from build123d import *

# Parameters (mm, degrees)
SKETCH3_R               = 27
SKETCH3_R_2             = 25
BOSS_EXTRUDE2_DEPTH     = 20
SKETCH4_W               = 21.394887062
SKETCH4_H               = 30
CUT_EXTRUDE1_DEPTH      = 28
CUT_EXTRUDE1_DEPTH_BACK = 28
SKETCH5_R               = 1.5
BOSS_EXTRUDE3_DEPTH     = 20
FILLET2_R               = 5
SKETCH6_R               = 32.5
BOSS_EXTRUDE4_DEPTH     = 3
SKETCH7_R               = 4
CUT_EXTRUDE2_DEPTH      = 4
SKETCH8_R               = 1.5
CUT_EXTRUDE3_DEPTH      = 4
CHAMFER1_SIZE           = 1
SKETCH9_R               = 3.5
BOSS_EXTRUDE5_DEPTH     = 30


with BuildPart() as part:
    # Sketch3 → Boss-Extrude2 (new body)
    with BuildSketch(Plane.XY):
        Circle(SKETCH3_R)
        Circle(SKETCH3_R_2, mode=Mode.SUBTRACT)
    extrude(amount=BOSS_EXTRUDE2_DEPTH)

    # Sketch4 → Cut-Extrude1 (cut, two sides)
    with BuildSketch(Plane(origin=(0, 0, 0), x_dir=(0, 0, -1), z_dir=(1, 0, 0))) as cut_extrude1_sk:
        with Locations((-13.697443531, 0)):
            Rectangle(SKETCH4_W, SKETCH4_H)
    extrude(amount=CUT_EXTRUDE1_DEPTH, mode=Mode.SUBTRACT)
    extrude(cut_extrude1_sk.sketch, amount=-CUT_EXTRUDE1_DEPTH_BACK, mode=Mode.SUBTRACT)

    # Sketch5 → Boss-Extrude3 (add)
    with BuildSketch(Plane.XY):
        with BuildLine():
            Line((-15.644487847, 19.5), (15.644487847, 19.5))
            ThreePointArc((15.644487847, 19.5), (0, 26.287924728), (-15.644487847, 19.5))
        make_face()
        with Locations((-7.5, 22.007101127)):
            Circle(SKETCH5_R, mode=Mode.SUBTRACT)
        with Locations((7.5, 22.007101127)):
            Circle(SKETCH5_R, mode=Mode.SUBTRACT)
        with BuildLine():
            ThreePointArc((8.529361055, -23.5), (0, -20.838962679), (-8.529361055, -23.5))
            ThreePointArc((-8.529361055, -23.5), (0, -26.208671307), (8.529361055, -23.5))
        make_face()
        with Locations((0, -23.25)):
            Circle(SKETCH5_R, mode=Mode.SUBTRACT)
    extrude(amount=BOSS_EXTRUDE3_DEPTH)

    # Fillet2
    fillet2_edges = [part.edges().sort_by_distance(p)[0] for p in [
        (15.644487847, 19.5, 10),
        (-15.644487847, 19.5, 10),
        (-8.529361055, -23.5, 10),
        (8.529361055, -23.5, 10),
    ]]
    fillet(fillet2_edges, radius=FILLET2_R)

    # Sketch6 → Boss-Extrude4 (add)
    with BuildSketch(Plane(origin=(0, 0, 0), x_dir=(-1, 0, 0), z_dir=(0, 0, -1))):
        Circle(SKETCH6_R)
    extrude(amount=-BOSS_EXTRUDE4_DEPTH)

    # Sketch7 → Cut-Extrude2 (cut, through all)
    with BuildSketch(Plane.XY.offset(3)):
        with Locations((0, 15)):
            Circle(SKETCH7_R)
    extrude(amount=-CUT_EXTRUDE2_DEPTH, mode=Mode.SUBTRACT)

    # Sketch8 → Cut-Extrude3 (cut, through all)
    with BuildSketch(Plane.XY.offset(3)):
        with Locations((-20, 0)):
            Circle(SKETCH8_R)
        with Locations((20, 0)):
            Circle(SKETCH8_R)
    extrude(amount=-CUT_EXTRUDE3_DEPTH, mode=Mode.SUBTRACT)

    # Chamfer1
    chamfer1_edges = [part.edges().sort_by_distance(p)[0] for p in [
        (-21.5, 0, 3),
        (18.5, 0, 3),
    ]]
    chamfer(chamfer1_edges, length=CHAMFER1_SIZE)

    # Sketch9 → Boss-Extrude5 (add)
    with BuildSketch(Plane.XY.offset(3)):
        with Locations((-12.35, -4)):
            Circle(SKETCH9_R)
        with Locations((12.35, -4)):
            Circle(SKETCH9_R)
    extrude(amount=BOSS_EXTRUDE5_DEPTH)


solid = part.part
Could you check a few things on this model? Use its own coordinates, in mm. A direction names the side the tool comes from. Round coordinates to 2 decimals unless told otherwise and drop trailing zeros. Write each loop counter-clockwise with the first axis right and the second up, starting at its lowest first coordinate (ties: lowest second). Pieces come first, ordered by that corner, then holes. Notation, with made-up numbers: (-23, 17) - (-1, 17) arc R35 cw to (-1, 56) - close; hole circle Ø4 at (66.5, 21). An arc over 180 degrees is marked (long way). Put each result on its own line as item: value. Start each with the question number.
(1) I want a section at A-A, the plane z = 23. Please give me the cut outline in (x, y), plus the area to 3 significant figures.
(2) I want a section at B-B, the plane z = 15. Give the number of separate pieces and of enclosed holes in the cut face, plus the area to 3 significant figures.
(3) I need wall thicknesses on probe 1 along Y at (x, z) = (15, 19); probe 2 along Z at (x, y) = (-18, -2); probe 3 along Y at (x, z) = (20, 0.8). Which ranges of each line are inside material? Lowest first, please.
(4) Will these pins go through, and if not, where does the flat tip stop? pin 1 (8.5 mm diameter, centred on x = -0.5, z = 7.5, fed in from -Y); pin 2 (0.7 mm diameter, centred on x = 21.5, z = 9, fed in from +Y); pin 3 (5 mm diameter, centred on x = 7.5, y = 22.01, fed in from -Z); pin 4 (4 mm diameter, centred on x = -13, z = 25.5, fed in from +Y).
(5) For faces 5 (the flat face through (0, 19.5, 11)), 6 (the flat face through (21, -15, 12)), 7 (the flat face through (0, 0, 0)), which set-ups out of +Z, -Z, +X, -X, +Y, -Y let a thin tool reach every point of the face, with its end or its side?
(6) Thinking about a two-plate mould opening in X: for faces 1 (the cylindrical face through (18.5, 0.07, 1.01)), 2 (the flat face through (-2, -22, 20)), 3 (the cylindrical face through (0, -27, 11)), 4 (the flat face through (-7, 22, 3)), which applies, released by +X, released by -X, zero draft, split by the parting line, or undercut?
Here are the results:
1. outline: circle Ø7 at (-12.35, -4); circle Ø7 at (12.35, -4)
1. area: 77.0 mm^2
2. separate pieces: 4
2. enclosed holes: 3
2. area: 423 mm^2
3. probe 1: y = -22.45 to -20, -6.29 to -1.71, 19.35 to 22.45
3. probe 2: z = 0 to 3
3. probe 3: y = -25.62 to -1.5, 1.5 to 25.62
4. pin 1: stops at y = -27
4. pin 2: stops at y = 16.78
4. pin 3: stops at z = 0
4. pin 4: stops at y = -0.5
5. face 5: +Z
5. face 6: +Z, +X, -X
5. face 7: -Z, +X, -X, +Y, -Y
6. face 1: undercut
6. face 2: zero draft
6. face 3: split by the parting line
6. face 4: undercut
